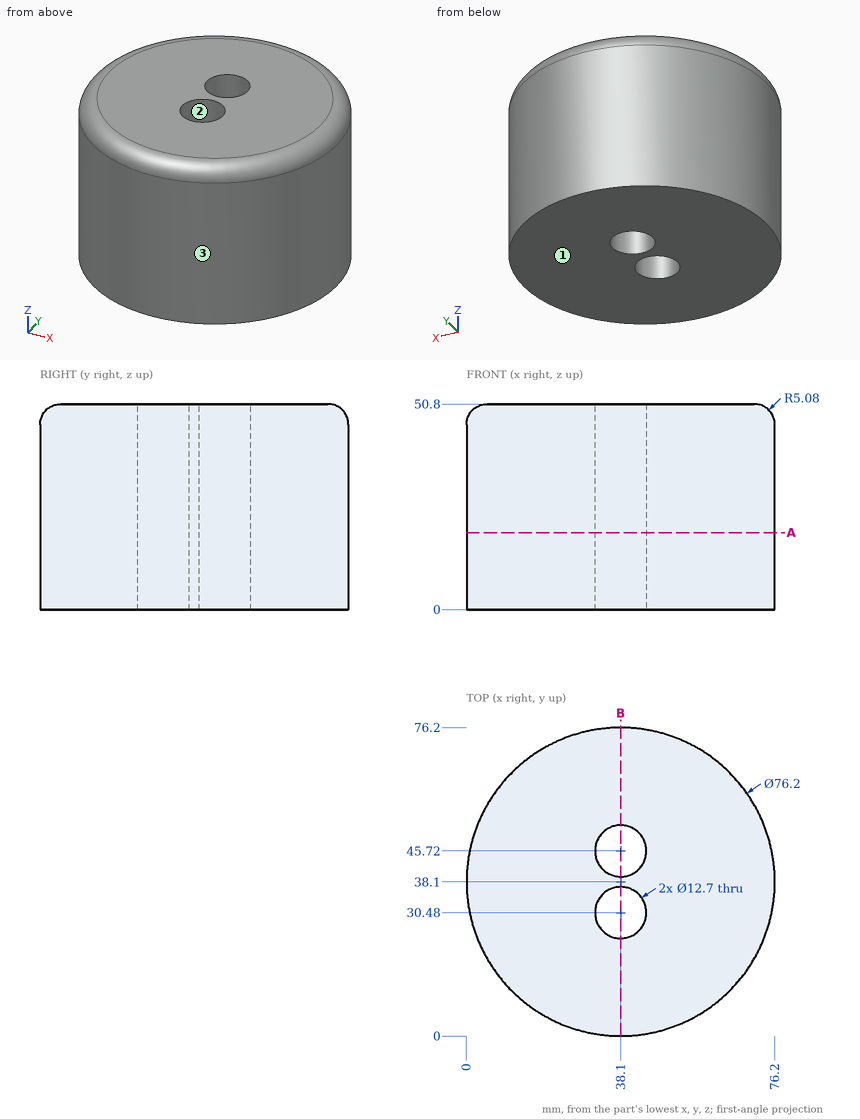
Geometry check sheet. Reference: drawing and pictorial views, mm from the part's lowest x, y, z. Round coordinates to 2 decimals unless told otherwise and drop trailing zeros. Write each loop counter-clockwise with the first axis right and the second up, starting at its lowest first coordinate (ties: lowest second). Pieces come first, ordered by that corner, then holes.
1. Gauge pin test, flat ends, axial feed: P1, Ø1, axis at x = 62, y = 13.5, coming from the +Z side; P2, Ø4, axis at y = 24, z = 6.5, coming from the +X side; P3, Ø2, axis at x = 47, z = 22.5, coming from the -Y side; P4, Ø10, axis at x = 38.1, y = 30.48, coming from the -Z side. Record the tip position at first contact, or that the pin passes through.
2. Section check A-A on z = 19. Enter the section's corners in (x, y), plus the area to 3 significant figures.
3. Scan lines: L1, parallel to Y at x = 38.1, z = 12; L2, parallel to Y at x = 35, z = 4; L3, parallel to X at y = 45, z = 40. Record each from-to range of solid material in increasing order.
4. Section check B-B on x = 38.1. State how many separate pieces and enclosed holes the cut face has, plus the area to 3 significant figures.
5. Draft check along Y on the marked faces 1, 2 and 3. Enter one of: +Y half, -Y half, draft (parallel to the pull), parting line (faces both ways), or undercut.
Answer:
1. P1: stops at z = 50.74
1. P2: stops at x = 74.23
1. P3: stops at y = 0.83
1. P4: passes through
2. outline: circle Ø76.2 at (38.1, 38.1); hole circle Ø12.7 at (38.1, 30.48); hole circle Ø12.7 at (38.1, 45.72)
2. area: 4,310 mm2
3. L1: y = 0 to 24.13, 36.83 to 39.37, 52.07 to 76.2
3. L2: y = 0.13 to 24.94, 36.02 to 40.18, 51.26 to 76.07
3. L3: x = 0.63 to 31.79, 44.41 to 75.57
4. separate pieces: 3
4. enclosed holes: 0
4. area: 2,570 mm2
5. face 1: draft
5. face 2: undercut
5. face 3: parting line
